Drawing for the job (mm, zero at the part's lowest x, y, z). Give positions to 0.01 mm unless a question says otherwise; leave off trailing zeros. Write each loop counter-clockwise with the first axis right and the second up, starting at its lowest first coordinate (ties: lowest second). Pieces come first, ordered by that corner, then holes. Notation, with made-up numbers: M -33.5,39.25 L 19.5,39.25 A23 ccw 19.5,50.25 Z; hole C 21,75 d7. An arc over 180 degrees is marked long. Answer as a JSON object with one key per item and string values. Group by question number.
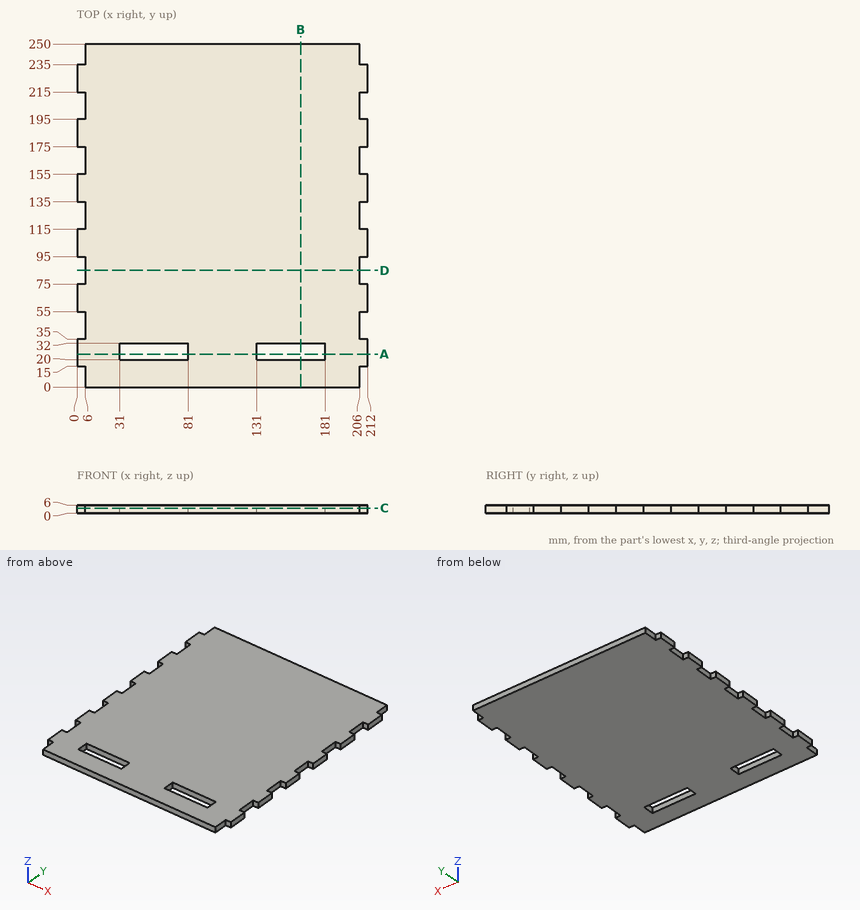
Q1. Slice it at A-A, the plane y = 24. Write the cut outline in (x, z).
Q2. Slice it at B-B, the plane x = 163. Write the cut outline in (y, z).
Q3. Drop flat-ended pins along their axis: P1, Ø3, axis at x = 2, z = 4, coming from the +Y side; P2, Ø1.8, axis at y = 239.5, z = 1.5, coming from the +X side; P3, Ø1.8, axis at x = 3.5, z = 3.5, coming from the -Y side. Give the stop position or say it passes through.
Q4. Slice it at D-D, the plane y = 85. Write the cut outline in (x, z), then the cut area to 3 significant figures.
Q5. Slice it at C-C, the plane z = 3.75. Count the separate pieces of the cut face and the enclosed holes in it, then the cut area to 3 significant figures.
Q6. Wall check: L1, parallel to Y at x = 145, z = 2.4; L2, parallel to X at y = 37, z = 3.3. Give the ranges that are in metal, low to high.
Solved:
{
 "1": {"outline": "M 0,0 L 31,0 L 31,6 L 0,6 Z; M 81,0 L 131,0 L 131,6 L 81,6 Z; M 181,0 L 212,0 L 212,6 L 181,6 Z"},
 "2": {"outline": "M 0,0 L 20,0 L 20,6 L 0,6 Z; M 32,0 L 250,0 L 250,6 L 32,6 Z"},
 "3": {"P1": "stops at y = 235", "P2": "stops at x = 206", "P3": "stops at y = 15"},
 "4": {"outline": "M 6,0 L 206,0 L 206,6 L 6,6 Z", "area": "1,200 mm²"},
 "5": {"separate pieces": "1", "enclosed holes": "2", "area": "50,200 mm²"},
 "6": {"L1": "y = 0 to 20, 32 to 250", "L2": "x = 6 to 206"}
}
